Model file for the job. Use its own axes, mm. Face numbers are marked on the shaded views. A direction names the side the tool comes from. Round coordinates to 2 decimals unless told otherwise and drop trailing zeros. Write each loop counter-clockwise with the first axis right and the second up, starting at its lowest first coordinate (ties: lowest second). Pieces come first, ordered by that corner, then holes. Notation, with made-up numbers: (11, 1.5) - (62, 1.5) arc R24 cw to (62, 33.5) - close; hole circle Ø3 at (18.5, 79.5). An arc over 180 degrees is marked (long way). Answer as a JSON object with one key per item and string values. Group by question number.
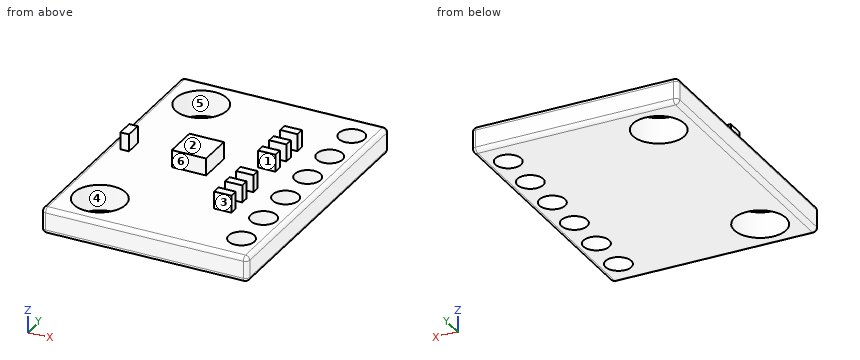
Autodesk Inventor part; units mm, degrees
ref_plane "YZ Plane" through (0, 0, 0) normal (1, 0, 0) x (0, 1, 0)
ref_plane "XZ Plane" through (0, 0, 0) normal (0, 1, 0) x (-1, 0, 0)
ref_plane "XY Plane" through (0, 0, 0) normal (0, 0, 1) x (1, 0, 0)
sketch "Szkic1" plane through (0, 0, 0) normal (0, 0, 1) x (1, 0, 0)
  point P0 (0, 0)
sketch "Szkic2" plane through (0, 0, 0) normal (0, 0, 1) x (1, 0, 0)
  line L0 (6, -8) -> (-6, -8)
  line L1 (-6, -8) -> (-6, 8)
  line L2 (-6, 8) -> (6, 8)
  line L3 (6, 8) -> (6, -8)
  line L4 (6, -8) -> (-6, 8) construction
  line L5 (-6, -8) -> (6, 8) construction
  point P0 (0, 0)
  dimension "d0" = 12
  dimension "d1" = 16
extrude "Wyciągnięcie proste1" add sketch "Szkic2" along normal blind 1.5
fillet "Zaokrąglenie1" radius 0.25 12 edges at (0, 8, 1.5) (0, 8, 0) (6, 0, 1.5) (6, 0, 0) (0, -8, 1.5) (0, -8, 0) (6, -8, 0.75) (6, 8, 0.75) (-6, 0, 1.5) (-6, 0, 0) (-6, -8, 0.75) (-6, 8, 0.75)
sketch "Szkic3" plane through (0, 0, 1.5) normal (0, 0, 1) x (1, 0, 0)
  line L0 (-5.75, -7.75) -> (-5.75, 7.75)
  line L1 (-5.75, -7.75) -> (-3.75, -7.75)
  line L2 (5.75, -7.75) -> (-5.75, -7.75)
  line L3 (-3.75, -7.75) -> (-3.75, -5.75)
  line L4 (-5.75, 7.75) -> (5.75, 7.75)
  line L5 (-5.75, 7.75) -> (-3.75, 7.75)
  line L6 (-3.75, 7.75) -> (-3.75, 5.75)
  line L7 (5.75, 7.75) -> (4.75, 7.75)
  line L8 (4.75, 7.75) -> (4.75, 6.25)
  line L9 (4.75, 6.25) -> (4.75, 3.75)
  line L10 (4.75, 3.75) -> (4.75, 1.25)
  line L11 (4.75, 1.25) -> (4.75, -1.25)
  line L12 (4.75, -1.25) -> (4.75, -3.75)
  line L13 (4.75, -3.75) -> (4.75, -6.25)
  circle A0 centre (-3.75, 5.75) radius 1.5
  circle A1 centre (-3.75, -5.75) radius 1.5
  circle A2 centre (4.75, -6.25) radius 0.5
  circle A3 centre (4.75, -3.75) radius 0.75
  circle A4 centre (4.75, -6.25) radius 0.75
  circle A5 centre (4.75, -1.25) radius 0.75
  circle A6 centre (4.75, 1.25) radius 0.75
  circle A7 centre (4.75, 3.75) radius 0.75
  circle A8 centre (4.75, 6.25) radius 0.75
  point P0 (0, 0)
  dimension "d5" = 2
  dimension "d6" = 2
  dimension "d7" = 2
  dimension "d8" = 2
  dimension "d9" = 1
  dimension "d10" = 1.5
  dimension "d11" = 2.5
  dimension "d12" = 2.5
  dimension "d13" = 2.5
  dimension "d14" = 2.5
  dimension "d15" = 2.5
  dimension "d17" = 3
  dimension "d18" = 3
  dimension "d19" = 1
  dimension "d20" = 1.5
  dimension "d21" = 1.5
  dimension "d22" = 1.5
  dimension "d23" = 1.5
  dimension "d24" = 1.5
  dimension "d25" = 1.5
extrude "Wyciągnięcie proste2" cut sketch "Szkic3" against normal blind 1.5 contours A2 | A4 | A3 L13 L12 | L12 L13 A3 | A5 L12 L11 | L11 L12 A5 | A6 L11 L10 | L10 L11 A6 | A7 L10 L9 | L9 L10 A7 | A8 L9 L8 | L8 L9 A8 | A0 | A1
sketch "Szkic4" plane through (0, 0, 1.5) normal (0, 0, 1) x (1, 0, 0)
  line L0 (3, -3.5) -> (2, -3.5)
  line L1 (2, -3.5) -> (2, -4)
  line L2 (2, -4) -> (3, -4)
  line L3 (3, -4) -> (3, -3.5)
  line L4 (3, -3.5) -> (2, -4) construction
  line L5 (2, -3.5) -> (3, -4) construction
  line L6 (3, -2.25) -> (2, -2.25)
  line L7 (2, -2.25) -> (2, -2.75)
  line L8 (2, -2.75) -> (3, -2.75)
  line L9 (3, -2.75) -> (3, -2.25)
  line L10 (3, -2.25) -> (2, -2.75) construction
  line L11 (2, -2.25) -> (3, -2.75) construction
  line L12 (3, -1) -> (2, -1)
  line L13 (2, -1) -> (2, -1.5)
  line L14 (2, -1.5) -> (3, -1.5)
  line L15 (3, -1.5) -> (3, -1)
  line L16 (3, -1) -> (2, -1.5) construction
  line L17 (2, -1) -> (3, -1.5) construction
  line L18 (3, 1.5) -> (2, 1.5)
  line L19 (2, 1.5) -> (2, 1)
  line L20 (2, 1) -> (3, 1)
  line L21 (3, 1) -> (3, 1.5)
  line L22 (3, 1.5) -> (2, 1) construction
  line L23 (2, 1.5) -> (3, 1) construction
  line L24 (3, 2.75) -> (2, 2.75)
  line L25 (2, 2.75) -> (2, 2.25)
  line L26 (2, 2.25) -> (3, 2.25)
  line L27 (3, 2.25) -> (3, 2.75)
  line L28 (3, 2.75) -> (2, 2.25) construction
  line L29 (2, 2.75) -> (3, 2.25) construction
  line L30 (3, 4) -> (2, 4)
  line L31 (2, 4) -> (2, 3.5)
  line L32 (2, 3.5) -> (3, 3.5)
  line L33 (3, 3.5) -> (3, 4)
  line L34 (3, 4) -> (2, 3.5) construction
  line L35 (2, 4) -> (3, 3.5) construction
  line L36 (-2, -1) -> (0, -1)
  line L37 (0, -1) -> (0, 1)
  line L38 (0, 1) -> (-2, 1)
  line L39 (-2, 1) -> (-2, -1)
  line L40 (-2, -1) -> (0, 1) construction
  line L41 (0, -1) -> (-2, 1) construction
  line L42 (-4.75, -0.5) -> (-5.25, -0.5)
  line L43 (-5.25, -0.5) -> (-5.25, 0.5)
  line L44 (-5.25, 0.5) -> (-4.75, 0.5)
  line L45 (-4.75, 0.5) -> (-4.75, -0.5)
  line L46 (-4.75, -0.5) -> (-5.25, 0.5) construction
  line L47 (-5.25, -0.5) -> (-4.75, 0.5) construction
  point P0 (0, 0)
  point P1 (2.5, -3.75)
  point P2 (2.5, -2.5)
  point P3 (2.5, -1.25)
  point P4 (2.5, 1.25)
  point P5 (2.5, 2.5)
  point P6 (2.5, 3.75)
  point P7 (-1, 0)
  point P8 (-5, 0)
  dimension "d28" = 1
  dimension "d29" = 0.5
  dimension "d30" = 1
extrude "Wyciągnięcie proste3" add sketch "Szkic4" along normal blind 1
properties part number "Czujnik BMP280"
(1) Flat gauge pins, fed straight in: pin 1 (0.8 mm diameter, centred on x = 2.5, z = 2, fed in from +Y); pin 2 (0.6 mm diameter, centred on y = 2.5, z = 2, fed in from +X); pin 3 (0.5 mm diameter, centred on x = 2.5, z = 2, fed in from -Y); pin 4 (0.9 mm diameter, centred on x = 4.75, y = -6.25, fed in from -Z). Where does each tip first touch, or does it go through?
(2) 3-axis set-ups, long thin cutter, end or side, ignore diameter. For the marked faces 5 and 6: which of +Z, -Z, +X, -X, +Y, -Y reach the whole face in a straight line?
(3) Drill centre lines: line 1 (X direction, y = -5.75, z = 0.75); line 2 (Z direction, x = 4.25, y = 2); line 3 (X direction, y = 5, z = 1.15). Where is each one in solid material? Low to high. Write a range as from..to.
(4) Slice it at D-D (y = 6). Write the cut outline in (x, z), then the cut area to 3 significant figures.
(5) Slice it at A-A (x = 4.75). Count the separate pieces of the cut face and the enclosed holes in it, then the cut area to 3 significant figures.
(6) Slice it at C-C (y = -3.75). Write the cut outline in (x, z).
(7) Pull direction Y, two halves, no side cores. Call the marked faces 1, 2, 3 and 4: pulls with the +Y half, pulls with the -Y half, needs draft (parallel to the pull), parting line crosses it, or undercut.
Answer:
{
 "1": {"pin 1": "y = 4", "pin 2": "x = 3", "pin 3": "y = -4", "pin 4": "through"},
 "2": {"face 5": "+Z, -Z", "face 6": "+Z, -X, -Y"},
 "3": {"line 1": "-6..-5.25, -2.25..4.19, 5.31..6", "line 2": "0..1.5", "line 3": "-6..-5.05, -2.45..6"},
 "4": {"outline": "(-6, 0.25) arc R0.25 ccw to (-5.75, 0) - (-5.23, 0) - (-5.23, 1.5) - (-5.75, 1.5) arc R0.25 ccw to (-6, 1.25) - close; (-2.27, 0) - (4.04, 0) - (4.04, 1.5) - (-2.27, 1.5) - close; (5.46, 0) - (5.75, 0) arc R0.25 ccw to (6, 0.25) - (6, 1.25) arc R0.25 ccw to (5.75, 1.5) - (5.46, 1.5) - close", "area": "11.4 mm²"},
 "5": {"separate pieces": "7", "enclosed holes": "0", "area": "10.4 mm²"},
 "6": {"outline": "(-6, 0.25) arc R0.25 ccw to (-5.75, 0) - (4, 0) - (4, 1.5) - (3, 1.5) - (3, 2.5) - (2, 2.5) - (2, 1.5) - (-5.75, 1.5) arc R0.25 ccw to (-6, 1.25) - close; (5.5, 0) - (5.75, 0) arc R0.25 ccw to (6, 0.25) - (6, 1.25) arc R0.25 ccw to (5.75, 1.5) - (5.5, 1.5) - close"},
 "7": {"face 1": "undercut", "face 2": "needs draft", "face 3": "pulls with the -Y half", "face 4": "undercut"}
}
